```python
from build123d import *

# Parameters (mm, degrees)
SKETCH1_R           = 2.25
BOSS_EXTRUDE1_DEPTH = 12


with BuildPart() as part:
    # Sketch1 → Boss-Extrude1 (new body)
    with BuildSketch(Plane(origin=(0, 0, 0), x_dir=(1, 0, 0), z_dir=(0, 1, 0))):
        Polygon((-23, 10), (-26, -10), (26, -10), (23, 10), align=None)
        with Locations((-12.75, 0)):
            Circle(SKETCH1_R, mode=Mode.SUBTRACT)
        with Locations((12.75, 0)):
            Circle(SKETCH1_R, mode=Mode.SUBTRACT)
    extrude(amount=BOSS_EXTRUDE1_DEPTH)


solid = part.part
```
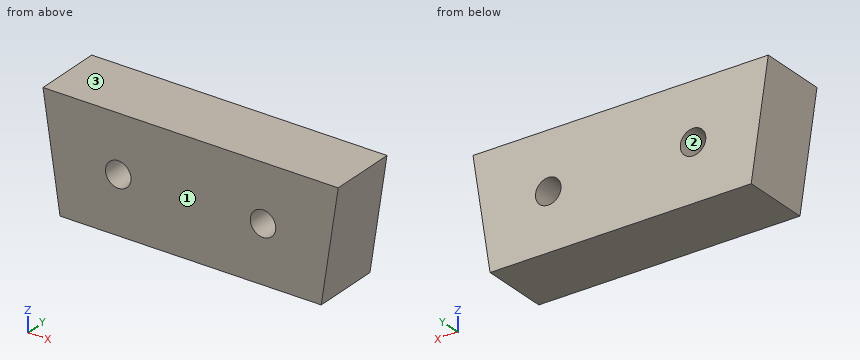
Can you work these out from the model? Positions are in its coordinate system, mm. Face numbers are marked on the shaded views. Coordinates: 2 decimals unless noted, no trailing zeros. Order: outer loops, then holes, each group sorted by start corner. A loop starts at its lowest first (then second) coordinate and runs counter-clockwise, first axis right, second up.
1. If we section it at C-C (y = 9): Please give me the cut outline in (x, z).
2. If we section it at B-B (x = 12.75): Please give me the cut outline in (y, z).
3. I need wall thicknesses on line 1 (Z direction, x = -12.75, y = 8.5); line 2 (X direction, y = 3, z = 1.25); line 3 (X direction, y = 3, z = 0). Which ranges of each line are inside material? Lowest first, please.
4. Thinking about a two-plate mould opening in Z: for the marked faces 1, 2 and 3, which applies, +Z half, -Z half, draft (parallel to the pull), parting line (faces both ways), or undercut?
5. I'm going to push flat-ended pins straight in: pin 1 (1.5 mm diameter, centred on y = 7.5, z = -2, fed in from +X); pin 2 (5 mm diameter, centred on y = 1, z = -3.5, fed in from -X). Where does each tip first touch, or does it pass through?
6. If we section it at A-A (z = 0): Please give me the cut outline in (x, y), then the cut area to 3 significant figures.
7. If we section it at D-D (z = -2.75): Please give me the cut outline in (x, y), then the cut area to 3 significant figures.
Entries:
1. outline: (-26, 10) - (-23, -10) - (23, -10) - (26, 10) - close; hole circle Ø4.5 at (-12.75, 0); hole circle Ø4.5 at (12.75, 0)
2. outline: (0, -10) - (12, -10) - (12, -2.25) - (0, -2.25) - close; (0, 2.25) - (12, 2.25) - (12, 10) - (0, 10) - close
3. line 1: z = -10 to -2.25, 2.25 to 10
3. line 2: x = -24.69 to -14.62, -10.88 to 10.88, 14.62 to 24.69
3. line 3: x = -24.5 to -15, -10.5 to 10.5, 15 to 24.5
4. face 1: draft
4. face 2: undercut
4. face 3: +Z half
5. pin 1: stops at x = 24.31
5. pin 2: stops at x = -24.35
6. outline: (-24.5, 0) - (-15, 0) - (-15, 12) - (-24.5, 12) - close; (-10.5, 0) - (10.5, 0) - (10.5, 12) - (-10.5, 12) - close; (15, 0) - (24.5, 0) - (24.5, 12) - (15, 12) - close
6. area: 480 mm2
7. outline: (-24.09, 0) - (24.09, 0) - (24.09, 12) - (-24.09, 12) - close
7. area: 578 mm2
